from build123d import *

# Parameters (mm, degrees)
CUT_EXTRUDE1_DEPTH = 2
CHAMFER1_SIZE      = 0.4


with BuildPart() as part:
    # Sketch1 → Revolve1 (revolve)
    with BuildSketch(Plane.XY, mode=Mode.PRIVATE) as revolve1_sk:
        Polygon((16, 0), (16, 2), (0, 2), (0, 3.5), (-2.8, 3.5), (-2.8, 0), align=None)
    revolve(revolve1_sk.sketch.rotate(Axis((-2.8, 0, 0), (1, 0, 0)), 90), axis=Axis((-2.8, 0, 0), (1, 0, 0)))

    # Sketch2 → Cut-Extrude1 (cut)
    with BuildSketch(Plane.ZY.offset(2.8)):
        Polygon((0, 1.732050808), (-1.5, 0.866025404), (-1.5, -0.866025404), (0, -1.732050808), (1.5, -0.866025404), (1.5, 0.866025404), align=None)
    extrude(amount=-CUT_EXTRUDE1_DEPTH, mode=Mode.SUBTRACT)

    # Sketch3 → Cut-Revolve1 (revolve, cut)
    with BuildSketch(Plane.XY, mode=Mode.PRIVATE) as cut_revolve1_sk:
        Polygon((0.066025404, 0), (-0.8, 1.5), (-0.8, 0), align=None)
    revolve(cut_revolve1_sk.sketch.rotate(Axis((-0.8, 0, 0), (1, 0, 0)), 90), axis=Axis((-0.8, 0, 0), (1, 0, 0)), mode=Mode.SUBTRACT)

    # Chamfer1
    chamfer1_edges = [part.edges().sort_by_distance(p)[0] for p in [
        (-2.8, 0, -3.5),
    ]]
    chamfer(chamfer1_edges, length=CHAMFER1_SIZE)


solid = part.part
The listing builds one solid part. Answer for the finished solid, in the listing's coordinates (mm). A direction names the side the tool comes from. Round coordinates to 2 decimals unless told otherwise and drop trailing zeros. Order: outer loops, then holes, each group sorted by start corner. A loop starts at its lowest first (then second) coordinate and runs counter-clockwise, first axis right, second up. Notation, with made-up numbers: (-38.5, 61.25) -> (-8.5, 61.25) arc R31 ccw to (-8.5, 88.25) -> close; hole circle Ø9 at (10.5, 6). An arc over 180 degrees is marked (long way). One line per item, written item: value.
Item 1: Find section A-A, the plane x = 3.5. Give the vertices of the cut face in (y, z), then the cut area to 3 significant figures.
Taken from the geometry:
outline: circle Ø4 at (0, 0)
area: 12.6 mm2
Item 2: Straight lines are drawn through the part: L1, parallel to Y at x = 3.25, z = -1; L2, parallel to X at y = -1.5, z = -0.25. For each, find the intervals that lie inside material, in ascending order.
Taken from the geometry:
L1: y = -1.73 to 1.73
L2: x = -0.8 to 16
Item 3: Given P1, Ø3, axis at x = 3, y = 0, coming from the +Z side; P2, Ø3, axis at x = -1, z = -2, coming from the +Y side, each flat-ended and moving along its own axis, determine where each tip first touches the part or whether it passes through.
Taken from the geometry:
P1: stops at z = 2
P2: stops at y = 3.46
Item 4: For faces 1 (the flat face through (0, 2, -2)), 2 (the cylindrical face through (-1.217, 3.105, 1.615)), 3 (the flat face through (-1.814, -1.305, 0.74)), determine the directions among +Z, -Z, +X, -X, +Y, -Y from which every point of the face is accessible in a straight line to the end or side of a thin tool.
Taken from the geometry:
face 1: +X
face 2: +X, -X
face 3: -X
